Work out the finished part from the listing and answer in its coordinate system (mm). Coordinates: 2 decimals unless noted, no trailing zeros. Write each loop counter-clockwise with the first axis right and the second up, starting at its lowest first coordinate (ties: lowest second). Pieces come first, ordered by that corner, then holes. Notation, with made-up numbers: M 68,65.25 L 88,65.25 A19 cw 88,90.25 Z; hole C 16,77.5 d11. An arc over 180 degrees is marked long. Use CSV: the item, a comma, the result in double quotes.
from build123d import *

# Parameters (mm, degrees)
F1_DEPTH = 0.75
F2_DEPTH = 0.75


# Not quite as in the source:
# - ends of sketch curves that miss each other by under 0.0002 mm in the source are joined


with BuildPart() as f1:
    # F0 (on Top) → F1 (new body)
    with BuildSketch(Plane.XY):
        with BuildLine():
            Line((-4.3542903055, 3.0103204122), (-15.1042902548, 3.0103204122))
            ThreePointArc((-15.1042902548, 3.0103204122), (-15.634620706, 2.7906503467), (-15.8542907714, 2.2603198956))
            Line((-15.8542907714, 2.2603198956), (-15.8542907714, -3.8396952234))
            ThreePointArc((-15.8542907714, -3.8396952234), (-15.634620706, -4.3700256746), (-15.1042902548, -4.58969574))
            Line((-15.1042902548, -4.58969574), (-6.6042903055, -4.58969574))
            Line((-6.6042903055, -4.58969574), (-6.6042903055, -3.8396876639))
            ThreePointArc((-6.6042903055, -3.8396876639), (-6.8239602196, -3.309357578), (-7.3542903055, -3.0896876639))
            Line((-7.3542903055, -3.0896876639), (-14.3542907714, -3.0896876639))
            Line((-14.3542907714, -3.0896876639), (-14.3542907714, 1.5103194803))
            Line((-14.3542907714, 1.5103194803), (-4.3542898395, 1.5103132679))
            ThreePointArc((-4.3542898395, 1.5103132679), (-3.8239600548, 1.2906431891), (-3.6042903055, 0.7603132679))
            Line((-3.6042903055, 0.7603132679), (-3.6042903055, -4.5896876639))
            Line((-3.6042903055, -4.5896876639), (-1.3042907714, -4.58969574))
            Line((-1.3042907714, -4.58969574), (-1.3042907714, -3.4706392285))
            ThreePointArc((-1.3042907714, -3.4706392285), (-1.3745455835, -3.153706188), (-1.5721480592, -2.8961492966))
            ThreePointArc((-1.5721480592, -2.8961492966), (-2.5098893785, -1.2818626098), (-2.2007190289, 0.5592495498))
            ThreePointArc((-2.2007190289, 0.5592495498), (-2.1287979009, 0.7369818479), (-2.1042903055, 0.9271417706))
            Line((-2.1042903055, 0.9271417706), (-2.1042903055, 3.7487632608))
            Line((-2.1042903055, 3.7487632608), (2.4957087627, 3.7487632608))
            Line((2.4957087627, 3.7487632608), (2.4957087627, 0.9271417706))
            ThreePointArc((2.4957087627, 0.9271417706), (2.5202163581, 0.7369818479), (2.5921374862, 0.5592495498))
            ThreePointArc((2.5921374862, 0.5592495498), (2.9013078357, -1.2818626098), (1.9635665164, -2.8961492966))
            ThreePointArc((1.9635665164, -2.8961492966), (1.7659640407, -3.153706188), (1.6957092286, -3.4706392285))
            Line((1.6957092286, -3.4706392285), (1.6957092286, -4.5896876639))
            Line((1.6957092286, -4.5896876639), (3.9957149822, -4.58969574))
            Line((3.9957149822, -4.58969574), (3.9957116586, 0.7603127188))
            ThreePointArc((3.9957116586, 0.7603127188), (4.2153814061, 1.290643318), (4.7457117418, 1.5103137014))
            Line((4.7457117418, 1.5103137014), (14.7457092286, 1.5103194803))
            Line((14.7457092286, 1.5103194803), (14.7457092286, -3.0896876639))
            Line((14.7457092286, -3.0896876639), (7.7457154989, -3.0896876639))
            ThreePointArc((7.7457154989, -3.0896876639), (7.2153850477, -3.3093577293), (6.9957149822, -3.8396881805))
            Line((6.9957149822, -3.8396881805), (6.9957149822, -4.5896876639))
            Line((6.9957149822, -4.5896876639), (15.495708712, -4.58969574))
            ThreePointArc((15.495708712, -4.58969574), (16.0260391632, -4.3700256746), (16.2457092286, -3.8396952234))
            Line((16.2457092286, -3.8396952234), (16.2457092286, 2.2603198956))
            ThreePointArc((16.2457092286, 2.2603198956), (16.0260391632, 2.7906503467), (15.495708712, 3.0103204122))
            Line((15.495708712, 3.0103204122), (4.7457149822, 3.0103204122))
            ThreePointArc((4.7457149822, 3.0103204122), (4.2153848964, 3.2299903263), (3.9957149822, 3.7603204122))
            Line((3.9957149822, 3.7603204122), (3.9957149822, 4.4987632608))
            ThreePointArc((3.9957149822, 4.4987632608), (3.7760450681, 5.0290933467), (3.2457149822, 5.2487632608))
            Line((3.2457149822, 5.2487632608), (-2.8542903055, 5.2487632608))
            ThreePointArc((-2.8542903055, 5.2487632608), (-3.3846203913, 5.0290933467), (-3.6042903055, 4.4987632608))
            Line((-3.6042903055, 4.4987632608), (-3.6042903055, 3.7603204122))
            ThreePointArc((-3.6042903055, 3.7603204122), (-3.8239602196, 3.2299903263), (-4.3542903055, 3.0103204122))
        make_face()
        with BuildLine():
            Line((-6.6042903055, -3.8396876639), (-6.6042903055, -4.58969574))
            Line((-6.6042903055, -4.58969574), (-3.6042903055, -4.58969574))
            Line((-3.6042903055, -4.58969574), (-3.6042903055, 0.7603132679))
            ThreePointArc((-3.6042903055, 0.7603132679), (-3.8239600548, 1.2906431891), (-4.3542898395, 1.5103132679))
            Line((-4.3542898395, 1.5103132679), (-14.3542907714, 1.5103194803))
            Line((-14.3542907714, 1.5103194803), (-14.3542907714, -3.0896876639))
            Line((-14.3542907714, -3.0896876639), (-7.3542903055, -3.0896876639))
            ThreePointArc((-7.3542903055, -3.0896876639), (-6.8239602196, -3.309357578), (-6.6042903055, -3.8396876639))
        make_face()
        with BuildLine():
            Line((3.9957116586, 0.7603127188), (3.9957149822, -4.5896876639))
            Line((3.9957149822, -4.5896876639), (6.9957149822, -4.58969574))
            Line((6.9957149822, -4.58969574), (6.9957149822, -3.8396881805))
            ThreePointArc((6.9957149822, -3.8396881805), (7.2153850477, -3.3093577293), (7.7457154989, -3.0896876639))
            Line((7.7457154989, -3.0896876639), (14.7457092286, -3.0896876639))
            Line((14.7457092286, -3.0896876639), (14.7457092286, 1.5103194803))
            Line((14.7457092286, 1.5103194803), (4.7457117418, 1.5103137014))
            ThreePointArc((4.7457117418, 1.5103137014), (4.2153814061, 1.290643318), (3.9957116586, 0.7603127188))
        make_face()
        with BuildLine():
            Line((-1.3042907714, -3.4706392285), (-1.3042907714, -4.5896876639))
            Line((-1.3042907714, -4.5896876639), (1.6957092286, -4.58969574))
            Line((1.6957092286, -4.58969574), (1.6957092286, -3.4706392285))
            ThreePointArc((1.6957092286, -3.4706392285), (1.7659640407, -3.153706188), (1.9635665164, -2.8961492966))
            ThreePointArc((1.9635665164, -2.8961492966), (2.9013078357, -1.2818626098), (2.5921374862, 0.5592495498))
            ThreePointArc((2.5921374862, 0.5592495498), (2.5202163581, 0.7369818479), (2.4957087627, 0.9271417706))
            Line((2.4957087627, 0.9271417706), (2.4957087627, 3.7487632608))
            Line((2.4957087627, 3.7487632608), (-2.1042903055, 3.7487632608))
            Line((-2.1042903055, 3.7487632608), (-2.1042903055, 0.9271417706))
            ThreePointArc((-2.1042903055, 0.9271417706), (-2.1287979009, 0.7369818479), (-2.2007190289, 0.5592495498))
            ThreePointArc((-2.2007190289, 0.5592495498), (-2.5098893785, -1.2818626098), (-1.5721480592, -2.8961492966))
            ThreePointArc((-1.5721480592, -2.8961492966), (-1.3745455835, -3.153706188), (-1.3042907714, -3.4706392285))
        make_face()
    extrude(amount=F1_DEPTH)

    # F0 (on Top) → F2 (join)
    with BuildSketch(Plane.XY):
        with BuildLine():
            Line((-6.6042903055, -3.8396876639), (-6.6042903055, -4.58969574))
            Line((-6.6042903055, -4.58969574), (-3.6042903055, -4.58969574))
            Line((-3.6042903055, -4.58969574), (-3.6042903055, 0.7603132679))
            ThreePointArc((-3.6042903055, 0.7603132679), (-3.8239600548, 1.2906431891), (-4.3542898395, 1.5103132679))
            Line((-4.3542898395, 1.5103132679), (-14.3542907714, 1.5103194803))
            Line((-14.3542907714, 1.5103194803), (-14.3542907714, -3.0896876639))
            Line((-14.3542907714, -3.0896876639), (-7.3542903055, -3.0896876639))
            ThreePointArc((-7.3542903055, -3.0896876639), (-6.8239602196, -3.309357578), (-6.6042903055, -3.8396876639))
        make_face()
        with BuildLine():
            Line((-1.3042907714, -3.4706392285), (-1.3042907714, -4.5896876639))
            Line((-1.3042907714, -4.5896876639), (1.6957092286, -4.58969574))
            Line((1.6957092286, -4.58969574), (1.6957092286, -3.4706392285))
            ThreePointArc((1.6957092286, -3.4706392285), (1.7659640407, -3.153706188), (1.9635665164, -2.8961492966))
            ThreePointArc((1.9635665164, -2.8961492966), (2.9013078357, -1.2818626098), (2.5921374862, 0.5592495498))
            ThreePointArc((2.5921374862, 0.5592495498), (2.5202163581, 0.7369818479), (2.4957087627, 0.9271417706))
            Line((2.4957087627, 0.9271417706), (2.4957087627, 3.7487632608))
            Line((2.4957087627, 3.7487632608), (-2.1042903055, 3.7487632608))
            Line((-2.1042903055, 3.7487632608), (-2.1042903055, 0.9271417706))
            ThreePointArc((-2.1042903055, 0.9271417706), (-2.1287979009, 0.7369818479), (-2.2007190289, 0.5592495498))
            ThreePointArc((-2.2007190289, 0.5592495498), (-2.5098893785, -1.2818626098), (-1.5721480592, -2.8961492966))
            ThreePointArc((-1.5721480592, -2.8961492966), (-1.3745455835, -3.153706188), (-1.3042907714, -3.4706392285))
        make_face()
        with BuildLine():
            Line((3.9957116586, 0.7603127188), (3.9957149822, -4.5896876639))
            Line((3.9957149822, -4.5896876639), (6.9957149822, -4.58969574))
            Line((6.9957149822, -4.58969574), (6.9957149822, -3.8396881805))
            ThreePointArc((6.9957149822, -3.8396881805), (7.2153850477, -3.3093577293), (7.7457154989, -3.0896876639))
            Line((7.7457154989, -3.0896876639), (14.7457092286, -3.0896876639))
            Line((14.7457092286, -3.0896876639), (14.7457092286, 1.5103194803))
            Line((14.7457092286, 1.5103194803), (4.7457117418, 1.5103137014))
            ThreePointArc((4.7457117418, 1.5103137014), (4.2153814061, 1.290643318), (3.9957116586, 0.7603127188))
        make_face()
    extrude(amount=-F2_DEPTH)


solid = f1.part
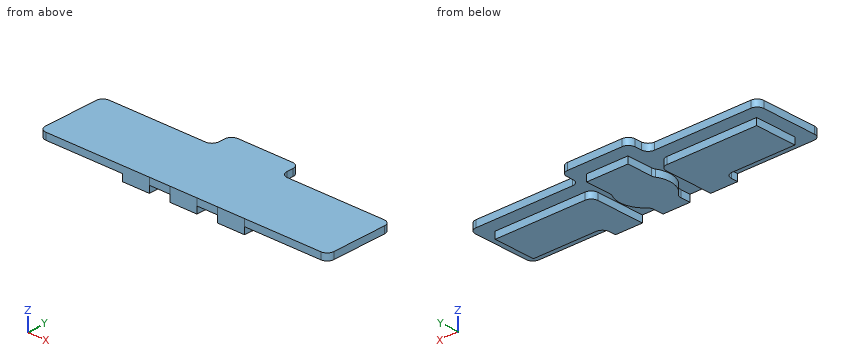
Item 1: Consider probe 1 along X at (y, z) = (-3.25, -0.05); probe 2 along X at (y, z) = (0, -0.45); probe 3 along Z at (x, y) = (4, 3.5). Determine where each line is inside the solid, lowest interval first.
Answer:
probe 1,"x = -6.89 to -3.6, -1.34 to 1.73, 4 to 7.28"
probe 2,"x = -14.35 to -3.6, -2.44 to 2.83, 4 to 14.75"
probe 3,"z = 0 to 0.75"
Item 2: The part is cut by section D-D (x = -13). Write down the section's boundary in (y, z).
Answer:
outline,"M -4.59,0 L -3.09,0 L -3.09,-0.75 L 1.51,-0.75 L 1.51,0 L 3.01,0 L 3.01,0.75 L -4.59,0.75 Z"
Item 3: Given pin 1 (0.6 mm diameter, centred on y = -4, z = -0.5, fed in from -X); pin 2 (0.8 mm diameter, centred on y = -1, z = -0.5, fed in from -X); pin 3 (0.6 mm diameter, centred on y = 3, z = -0.5, fed in from -X), each flat-ended and moving along its own axis, determine where each tip first touches the part or whether it passes through.
Answer:
pin 1,"stops at x = -6.62"
pin 2,"stops at x = -14.35"
pin 3,"stops at x = -2.1"
Item 4: The part is cut by section C-C (y = -1.25). Write down the section's boundary in (x, z).
Answer:
outline,"M -15.85,0 L -14.35,0 L -14.35,-0.75 L -3.6,-0.75 L -3.6,0 L -2.52,0 L -2.52,-0.75 L 2.91,-0.75 L 2.91,0 L 4,0 L 4,-0.75 L 14.75,-0.75 L 14.75,0 L 16.25,0 L 16.25,0.75 L -15.85,0.75 Z"
Item 5: The part is cut by section A-A (z = -0.45). Write down the section's boundary in (x, y), then the cut area to 3 significant figures.
Answer:
outline,"M -14.35,-3.09 L -7.35,-3.09 A0.75 cw -6.6,-3.84 L -6.6,-4.59 L -3.6,-4.59 L -3.6,0.76 A0.75 ccw -4.35,1.51 L -14.35,1.51 Z; M -2.2,0.56 A2.75 ccw -1.57,-2.9 A0.75 cw -1.3,-3.47 L -1.3,-4.59 L 1.7,-4.59 L 1.7,-3.47 A0.75 cw 1.96,-2.9 A2.75 ccw 2.59,0.56 A0.75 cw 2.5,0.93 L 2.5,3.75 L -2.1,3.75 L -2.1,0.93 A0.75 cw Z; M 4,-4.59 L 7,-4.59 L 7,-3.84 A0.75 cw 7.75,-3.09 L 14.75,-3.09 L 14.75,1.51 L 4.75,1.51 A0.75 ccw 4,0.76 Z"
area,"145 mm2"
Item 6: The part is cut by section B-B (x = 1). Write down the section's boundary in (y, z), then the cut area to 3 significant figures.
Answer:
outline,"M -4.59,-0.75 L 3.75,-0.75 L 3.75,0 L 5.25,0 L 5.25,0.75 L -4.59,0.75 Z"
area,"13.6 mm2"
